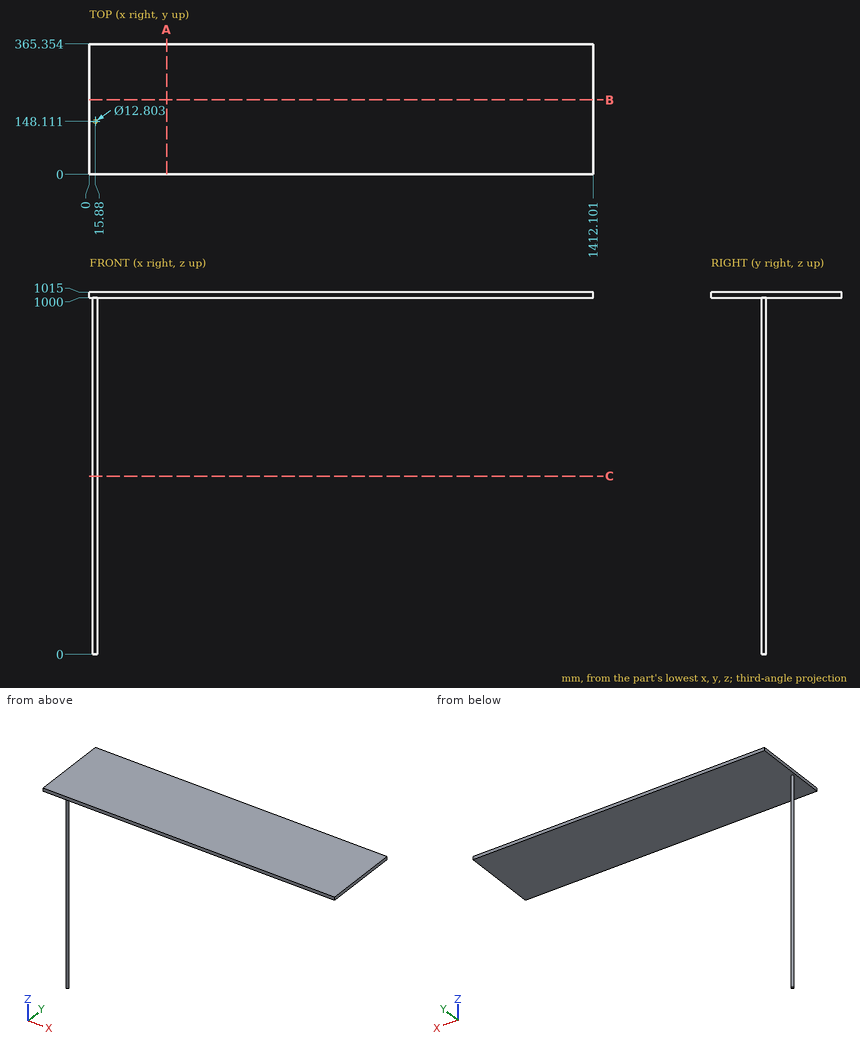
The figure shows three views and two pictorial views of one solid part (mm, origin at its lowest corner). Answer the questions. Coordinates: 2 decimals unless noted, no trailing zeros. Loops run counter-clockwise (first coordinate to the right, second up) from the corner with the lowest first, then second, coordinate; pieces in that order, holes last.
(1) The part is cut by section B-B (y = 208.5). Determine the outline of the cut face in (x, z), and give its area (3 significant figures).
Solution:
outline: (0, 1000) - (1412.1, 1000) - (1412.1, 1015) - (0, 1015) - close
area: 21,200 mm2
(2) A flat-ended cylindrical pin translates along its axis: pin 1 Ø5 at (x, y) = (303, 233.5) entering from -Z. Find the tip coordinate at first contact, or state that the pin passes through.
Solution:
pin 1: stops at z = 1000
(3) Consider line 1 along Z through (x, y) = (826, 90). Determine where the line is inside the solid, lowest interval first.
Solution:
line 1: z = 1000 to 1015
(4) The part is cut by section C-C (z = 500). Determine the outline of the cut face in (x, y).
Solution:
outline: circle Ø12.8 at (15.88, 148.11)
(5) The part is cut by section A-A (x = 216.5). Determine the outline of the cut face in (y, z).
Solution:
outline: (0, 1000) - (365.35, 1000) - (365.35, 1015) - (0, 1015) - close
